from build123d import *

# Parameters (mm, degrees)
SKETCH1_W                                      = 83.058
SKETCH1_H                                      = 82.55
BOSS_EXTRUDE1_DEPTH                            = 2.794
SKETCH2_W                                      = 58.7375
SKETCH2_H                                      = 42.9895
SKETCH2_W_2                                    = 54.9275
SKETCH2_H_2                                    = 39.1795
BOSS_EXTRUDE2_DEPTH                            = 11.1125
SKETCH5_W                                      = 66.929
SKETCH5_H                                      = 49.403
CUT_EXTRUDE1_DEPTH                             = 1.27
SKETCH2_2_W                                    = 54.9275
SKETCH2_2_H                                    = 39.1795
CUT_EXTRUDE2_DEPTH                             = 60.596737513
CSK_FOR_2_FLAT_HEAD_MACHINE_SCREW1_D           = 2.4384
CSK_FOR_2_FLAT_HEAD_MACHINE_SCREW1_CSINK_D     = 4.8104044
CSK_FOR_2_FLAT_HEAD_MACHINE_SCREW1_CSINK_ANGLE = 82
SKETCH9_W                                      = 12.7
SKETCH9_H                                      = 2.54
CUT_EXTRUDE4_DEPTH                             = 9.8044
SKETCH10_W                                     = 12.7
SKETCH10_H                                     = 3.048
CUT_EXTRUDE5_DEPTH                             = 0.254
SKETCH11_W                                     = 3.175
SKETCH11_H                                     = 9.525
CUT_EXTRUDE7_DEPTH                             = 1.524
SKETCH12_W                                     = 2.032
SKETCH12_H                                     = 19.05
CUT_EXTRUDE8_DEPTH                             = 82.161030266
SKETCH14_W                                     = 3.175
SKETCH14_H                                     = 19.05
CUT_EXTRUDE11_DEPTH                            = 0.508
FILLET2_R                                      = 4.7625
SKETCH15_W                                     = 54.9275
SKETCH15_H                                     = 1.905
CUT_EXTRUDE12_DEPTH                            = 8.3185
SKETCH16_W                                     = 54.9275
SKETCH16_H                                     = 1.524
CUT_EXTRUDE13_DEPTH                            = 1.5875
SKETCH17_W                                     = 12.7
SKETCH17_H                                     = 2.6543
BOSS_EXTRUDE3_DEPTH                            = 0.1016
SKETCH18_W                                     = 12.7
SKETCH18_H                                     = 0.3556
CUT_EXTRUDE14_DEPTH                            = 0.1016
SKETCH19_W                                     = 161.493776118
SKETCH19_H                                     = 133.946930056
SKETCH19_W_2                                   = 82.55
SKETCH19_H_2                                   = 82.042
CUT_EXTRUDE15_DEPTH                            = 60.596737513
FILLET3_R                                      = 1.5875
SKETCH21_W                                     = 80.9625
SKETCH21_H                                     = 3.175
BOSS_EXTRUDE4_DEPTH                            = 9.906
SKETCH22_W                                     = 19.05
SKETCH22_H                                     = 9.525
BOSS_EXTRUDE5_DEPTH                            = 3.175
SKETCH23_W                                     = 12.7
SKETCH23_H                                     = 1.016
CUT_EXTRUDE16_DEPTH                            = 7.8994
SKETCH24_R                                     = 2.60985
CUT_EXTRUDE17_DEPTH                            = 67.163598214
SKETCH25_W                                     = 80.9625
SKETCH25_H                                     = 3.175
CUT_EXTRUDE18_DEPTH                            = 0.254
CHAMFER1_SIZE                                  = 1.016
CUT_EXTRUDE19_DEPTH                            = 60.255810196
SKETCH29_W                                     = 54.9275
SKETCH29_H                                     = 4.1021
CUT_EXTRUDE20_DEPTH                            = 0.381
CHAMFER2_SIZE                                  = 0.508


with BuildPart() as part:
    # Sketch1 → Boss-Extrude1 (new body)
    with BuildSketch(Plane.XY):
        Rectangle(SKETCH1_W, SKETCH1_H)
    extrude(amount=BOSS_EXTRUDE1_DEPTH)

    # Sketch2 → Boss-Extrude2 (add)
    with BuildSketch(Plane(origin=(0, 0, 0), x_dir=(-1, 0, 0), z_dir=(0, 0, -1))):
        with Locations((0, -15.56385)):
            Rectangle(SKETCH2_W, SKETCH2_H)
        with Locations((0, -15.56385)):
            Rectangle(SKETCH2_W_2, SKETCH2_H_2, mode=Mode.SUBTRACT)
    extrude(amount=-BOSS_EXTRUDE2_DEPTH)

    # Sketch5 → Cut-Extrude1 (cut)
    with BuildSketch(Plane(origin=(0, 0, 0), x_dir=(-1, 0, 0), z_dir=(0, 0, -1))):
        with Locations((0, -16.5735)):
            Rectangle(SKETCH5_W, SKETCH5_H)
    extrude(amount=-CUT_EXTRUDE1_DEPTH, mode=Mode.SUBTRACT)

    # Sketch2<2> → Cut-Extrude2 (cut, through all)
    with BuildSketch(Plane(origin=(0, 0, 0), x_dir=(-1, 0, 0), z_dir=(0, 0, -1))):
        with Locations((0, -15.56385)):
            Rectangle(SKETCH2_2_W, SKETCH2_2_H)
    extrude(amount=-CUT_EXTRUDE2_DEPTH, mode=Mode.SUBTRACT)

    # CSK for #2 Flat Head Machine Screw1 (through all)
    with Locations(Plane(origin=(0, 0, 0), x_dir=(-1, 0, 0), z_dir=(0, 0, -1))):
        with Locations((37.592, 37.211), (-37.592, 37.211), (-37.592, -37.211), (37.592, -37.211)):
            CounterSinkHole(CSK_FOR_2_FLAT_HEAD_MACHINE_SCREW1_D / 2, CSK_FOR_2_FLAT_HEAD_MACHINE_SCREW1_CSINK_D / 2, counter_sink_angle=CSK_FOR_2_FLAT_HEAD_MACHINE_SCREW1_CSINK_ANGLE)

    # Sketch9 → Cut-Extrude4 (cut)
    with BuildSketch(Plane.XZ.offset(-4.0259)):
        with Locations((0, 2.54)):
            Rectangle(SKETCH9_W, SKETCH9_H)
    extrude(amount=-CUT_EXTRUDE4_DEPTH, mode=Mode.SUBTRACT)

    # Sketch10 → Cut-Extrude5 (cut)
    with BuildSketch(Plane.XY.offset(1.27)):
        with Locations((0, 12.3063)):
            Rectangle(SKETCH10_W, SKETCH10_H)
    extrude(amount=-CUT_EXTRUDE5_DEPTH, mode=Mode.SUBTRACT)

    # Sketch11 → Cut-Extrude7 (cut)
    with BuildSketch(Plane(origin=(0, 0, 1.27), x_dir=(-1, 0, 0), z_dir=(0, 0, -1))):
        with Locations((-29.05125, -25.2095)):
            Rectangle(SKETCH11_W, SKETCH11_H)
    cut_extrude7 = extrude(amount=-CUT_EXTRUDE7_DEPTH, mode=Mode.SUBTRACT)

    # Sketch12 → Cut-Extrude8 (cut, through all)
    with BuildSketch(Plane.ZY.offset(-27.46375)):
        with Locations((3.81, -20.447)):
            Rectangle(SKETCH12_W, SKETCH12_H)
    cut_extrude8 = extrude(amount=-CUT_EXTRUDE8_DEPTH, mode=Mode.SUBTRACT)

    # Sketch14 → Cut-Extrude11 (cut)
    with BuildSketch(Plane.XY.offset(2.794)):
        with Locations((29.05125, -20.447)):
            Rectangle(SKETCH14_W, SKETCH14_H)
    cut_extrude11 = extrude(amount=-CUT_EXTRUDE11_DEPTH, mode=Mode.SUBTRACT)

    # Mirror1: Cut-Extrude7, Cut-Extrude8, Cut-Extrude11 across plane
    add(cut_extrude7.mirror(Plane(origin=(0, 0, 0), x_dir=(0, 0, 1), z_dir=(1, 0, 0))), mode=Mode.SUBTRACT)
    add(cut_extrude8.mirror(Plane(origin=(0, 0, 0), x_dir=(0, 0, 1), z_dir=(1, 0, 0))), mode=Mode.SUBTRACT)
    add(cut_extrude11.mirror(Plane(origin=(0, 0, 0), x_dir=(0, 0, 1), z_dir=(1, 0, 0))), mode=Mode.SUBTRACT)

    # Fillet2
    fillet2_edges = [part.edges().sort_by_distance(p)[0] for p in [
        (-33.4645, 8.128, 0.635),
        (33.4645, 8.128, 0.635),
    ]]
    fillet(fillet2_edges, radius=FILLET2_R)

    # Sketch15 → Cut-Extrude12 (cut)
    with BuildSketch(Plane.XY.offset(11.1125)):
        with Locations((0, -36.1061)):
            Rectangle(SKETCH15_W, SKETCH15_H)
    extrude(amount=-CUT_EXTRUDE12_DEPTH, mode=Mode.SUBTRACT)

    # Sketch16 → Cut-Extrude13 (cut)
    with BuildSketch(Plane(origin=(0, -35.1536, 0), x_dir=(1, 0, 0), z_dir=(0, 1, 0))):
        with Locations((0, -2.032)):
            Rectangle(SKETCH16_W, SKETCH16_H)
    extrude(amount=-CUT_EXTRUDE13_DEPTH, mode=Mode.SUBTRACT)

    # Sketch17 → Boss-Extrude3 (add)
    with BuildSketch(Plane.XY.offset(1.27)):
        with Locations((0, 9.45515)):
            Rectangle(SKETCH17_W, SKETCH17_H)
    extrude(amount=BOSS_EXTRUDE3_DEPTH)

    # Sketch18 → Cut-Extrude14 (cut)
    with BuildSketch(Plane(origin=(0, 10.7823, 0), x_dir=(1, 0, 0), z_dir=(0, 1, 0))):
        with Locations((0, -1.1938)):
            Rectangle(SKETCH18_W, SKETCH18_H)
    extrude(amount=-CUT_EXTRUDE14_DEPTH, mode=Mode.SUBTRACT)

    # Sketch19 → Cut-Extrude15 (cut, through all)
    with BuildSketch(Plane(origin=(0, 0, 0), x_dir=(-1, 0, 0), z_dir=(0, 0, -1))):
        Rectangle(SKETCH19_W, SKETCH19_H)
        Rectangle(SKETCH19_W_2, SKETCH19_H_2, mode=Mode.SUBTRACT)
    extrude(amount=-CUT_EXTRUDE15_DEPTH, mode=Mode.SUBTRACT)

    # Fillet3
    fillet3_edges = [part.edges().sort_by_distance(p)[0] for p in [
        (41.275, 41.021, 1.397),
        (-41.275, 41.021, 1.397),
        (-41.275, -41.021, 1.397),
        (41.275, -41.021, 1.397),
    ]]
    fillet(fillet3_edges, radius=FILLET3_R)

    # Sketch21 → Boss-Extrude4 (add)
    with BuildSketch(Plane.XY.offset(2.794)):
        with Locations((0, 10.6934)):
            Rectangle(SKETCH21_W, SKETCH21_H)
    extrude(amount=BOSS_EXTRUDE4_DEPTH)

    # Sketch22 → Boss-Extrude5 (add)
    with BuildSketch(Plane.XY.offset(2.794)):
        with Locations((0, 10.6934)):
            Rectangle(SKETCH22_W, SKETCH22_H)
    extrude(amount=BOSS_EXTRUDE5_DEPTH)

    # Sketch23 → Cut-Extrude16 (cut)
    with BuildSketch(Plane.XZ.offset(-5.9309)):
        with Locations((0, 3.302)):
            Rectangle(SKETCH23_W, SKETCH23_H)
    extrude(amount=-CUT_EXTRUDE16_DEPTH, mode=Mode.SUBTRACT)

    # Sketch24 → Cut-Extrude17 (cut, through all)
    with BuildSketch(Plane.XZ.offset(-9.1059)):
        with Locations((-31.5, 12.7)):
            Circle(SKETCH24_R)
        with Locations((-22.5, 12.7)):
            Circle(SKETCH24_R)
        with Locations((31.5, 12.7)):
            Circle(SKETCH24_R)
        with Locations((22.5, 12.7)):
            Circle(SKETCH24_R)
        with Locations((13.5, 12.7)):
            Circle(SKETCH24_R)
        with Locations((4.5, 12.7)):
            Circle(SKETCH24_R)
        with Locations((-4.5, 12.7)):
            Circle(SKETCH24_R)
        with Locations((-13.5, 12.7)):
            Circle(SKETCH24_R)
    extrude(amount=-CUT_EXTRUDE17_DEPTH, mode=Mode.SUBTRACT)

    # Sketch25 → Cut-Extrude18 (cut)
    with BuildSketch(Plane.XY.offset(12.7)):
        with Locations((0, 10.6934)):
            Rectangle(SKETCH25_W, SKETCH25_H)
    extrude(amount=-CUT_EXTRUDE18_DEPTH, mode=Mode.SUBTRACT)

    # Chamfer1
    chamfer1_edges = [part.edges().sort_by_distance(p)[0] for p in [
        (-40.48125, 10.6934, 12.446),
        (40.48125, 10.6934, 12.446),
    ]]
    chamfer(chamfer1_edges, length=CHAMFER1_SIZE)

    # Sketch26 → Cut-Extrude19 (cut, through all)
    with BuildSketch(Plane(origin=(0, 0, 1.27), x_dir=(-1, 0, 0), z_dir=(0, 0, -1))):
        with BuildLine():
            Line((-28.2575, -23.45055), (-28.2575, -25.06345))
            ThreePointArc((-28.2575, -25.06345), (-29.845, -26.65095), (-31.4325, -25.06345))
            Line((-31.4325, -25.06345), (-31.4325, -23.45055))
            ThreePointArc((-31.4325, -23.45055), (-29.845, -21.86305), (-28.2575, -23.45055))
        make_face()
    extrude(amount=-CUT_EXTRUDE19_DEPTH, mode=Mode.SUBTRACT)

    # Sketch29 → Cut-Extrude20 (cut)
    with BuildSketch(Plane(origin=(0, 0, 1.27), x_dir=(-1, 0, 0), z_dir=(0, 0, -1))):
        with Locations((0, 6.07695)):
            Rectangle(SKETCH29_W, SKETCH29_H)
    extrude(amount=-CUT_EXTRUDE20_DEPTH, mode=Mode.SUBTRACT)

    # Chamfer2
    chamfer2_edges = [part.edges().sort_by_distance(p)[0] for p in [
        (-16.906875, 4.0259, 1.651),
        (16.906875, 4.0259, 1.651),
    ]]
    chamfer(chamfer2_edges, length=CHAMFER2_SIZE)


solid = part.part
Work out the finished part from the listing and answer in its coordinate system (mm). A direction names the side the tool comes from. Coordinates: 2 decimals unless noted, no trailing zeros. Loops run counter-clockwise (first coordinate to the right, second up) from the corner with the lowest first, then second, coordinate; pieces in that order, holes last. Notation, with made-up numbers: M 86.25,79.5 L 123.25,79.5 A21 cw 123.25,95.5 Z; hole C -29,43.25 d8. An arc over 180 degrees is marked long. Answer in a Markdown table with one row per item. Add a question column.
1. Find section B-B, the plane x = 0. Write down the section's boundary in (y, z).
2. Find section D-D, the plane y = 24. Write down the section's boundary in (x, z) (3 decimals).
3. Flat-ended cylindrical pins translate along their axes: P1, Ø3, axis at x = 14.5, y = 6, coming from the -Z side; P2, Ø4, axis at x = -37.592, y = 37.211, coming from the -Z side; P3, Ø5, axis at x = 13.5, z = 8, coming from the +Y side. Find the tip coordinate at first contact, or state that the pin passes through.
4. A tool of negligible diameter and unlimited length cuts with its end or side. For faces 5 (the flat face through (9.525, 14, 4)), 6 (the cylindrical face through (13.45, 10.67, 10.09)), 7 (the flat face through (29.369, -32, 7)), from which of +Z, -Z, +X, -X, +Y, -Y can it reach the whole face along a straight path? Write none if from no direction.
5. Find section C-C, the plane x = 15. Write down the section's boundary in (y, z), then the cut area to 3 significant figures.
6. The mould has two halves that part along Y. Classify faces 1 (the cylindrical face through (-13.55, 10.67, 10.09)), 2 (the flat face through (-29, -10.922, 3)), 3 (the cylindrical face through (-32.1, 6.7, 0.6)), 4 (the flat face through (0, 12, 1.016)): pulls with the +Y half, pulls with the -Y half, needs draft (parallel to the pull), parting line crosses it, or undercut.
7. Consider L1, parallel to Y at x = -27.5, z = 4; L2, parallel to Y at x = -20.5, z = 10.25; L3, parallel to Y at x = 7, z = 2.5. Determine where each line is inside the solid, lowest interval first.
8. Find section A-A, the plane y = -19.5. Write down the section's boundary in (x, z) (1 decimal), then the cut area to 3 significant figures.
Reported:
| question | item | result |
|---|---|---|
| 1 | outline | M -41.02,1.27 L -36.74,1.27 L -36.74,2.79 L -41.02,2.79 Z; M 4.03,3.81 L 13.83,3.81 L 13.83,1.02 L 10.68,1.02 L 10.68,1.37 L 8.13,1.37 L 8.13,0 L 41.02,0 L 41.02,2.79 L 15.46,2.79 L 15.46,5.97 L 12.28,5.97 L 12.28,12.45 L 9.11,12.45 L 9.11,5.97 L 5.93,5.97 L 5.93,11.11 L 4.03,11.11 Z |
| 2 | outline | M -41.275,0 L 41.275,0 L 41.275,2.794 L -41.275,2.794 Z |
| 3 | P1 | stops at z = 1.65 |
| 3 | P2 | stops at z = 0.47 |
| 3 | P3 | stops at y = 12.28 |
| 4 | face 5 | +Z, +X, +Y |
| 4 | face 6 | +Z, +Y |
| 4 | face 7 | +Z, +X, -Y |
| 5 | outline | M -41.02,1.27 L -36.74,1.27 L -36.74,2.79 L -41.02,2.79 Z; M 4.03,2.16 L 4.53,1.65 L 8.13,1.65 L 8.13,0 L 41.02,0 L 41.02,2.79 L 12.28,2.79 L 12.28,10.56 L 9.11,10.56 L 9.11,2.79 L 5.93,2.79 L 5.93,11.11 L 4.03,11.11 Z |
| 5 | area | 144 mm^2 |
| 6 | face 1 | needs draft |
| 6 | face 2 | undercut |
| 6 | face 3 | pulls with the -Y half |
| 6 | face 4 | undercut |
| 7 | L1 | y = -37.06 to -29.97, -10.92 to 5.93, 9.11 to 12.28 |
| 7 | L2 | y = 4.03 to 5.93, 9.11 to 12.28 |
| 7 | L3 | y = -41.02 to -36.74, 4.03 to 41.02 |
| 8 | outline | M -41.3,0 L -33.5,0 L -33.5,1.3 L -27.5,1.3 L -27.5,2.3 L -30.6,2.3 L -30.6,2.8 L -41.3,2.8 Z; M -29.4,4.8 L -27.5,4.8 L -27.5,11.1 L -29.4,11.1 Z; M 27.5,1.3 L 33.5,1.3 L 33.5,0 L 41.3,0 L 41.3,2.8 L 30.6,2.8 L 30.6,2.3 L 27.5,2.3 Z; M 27.5,4.8 L 29.4,4.8 L 29.4,11.1 L 27.5,11.1 Z |
| 8 | area | 82.7 mm^2 |
